The listing builds one solid part. Answer for the finished solid, in the listing's coordinates (mm). A direction names the side the tool comes from. Coordinates: 2 decimals unless noted, no trailing zeros. Order: outer loops, then holes, each group sorted by start corner. A loop starts at its lowest first (then second) coordinate and runs counter-clockwise, first axis right, second up. Notation, with made-up numbers: (39, 48.25) - (90, 48.25) arc R14 cw to (90, 74.25) - close; hole circle Ø11 at (23, 45). An arc over 180 degrees is marked (long way). One line per item, written item: value. Start each with the question number.
```python
from build123d import *

# Parameters (mm, degrees)
SKETCH1_W           = 10
SKETCH1_H           = 26
BOSS_EXTRUDE1_DEPTH = 15
SKETCH2_R           = 5
BOSS_EXTRUDE2_DEPTH = 20


with BuildPart() as part:
    # Sketch1 → Boss-Extrude1 (new body)
    with BuildSketch(Plane.XY):
        Rectangle(SKETCH1_W, SKETCH1_H)
    extrude(amount=BOSS_EXTRUDE1_DEPTH)

    # Sketch2 → Boss-Extrude2 (add)
    with BuildSketch(Plane.XY.offset(15)):
        Circle(SKETCH2_R)
    extrude(amount=BOSS_EXTRUDE2_DEPTH)

    # Sketch3 → Revolve1 (revolve)
    with BuildSketch(Plane.XY.offset(35)):
        with BuildLine():
            Line((-7, 0), (7, 0))
            ThreePointArc((7, 0), (0, 7), (-7, 0))
        make_face()
    revolve(axis=Axis((-7, 0, 35), (1, 0, 0)))


solid = part.part
```
(1) Consider probe 1 along Z at (x, y) = (1.5, -9.5); probe 2 along X at (y, z) = (7.75, 9.5); probe 3 along Z at (x, y) = (-4, 3.25). Determine where each line is inside the solid, lowest interval first.
(2) The part is cut by section B-B on y = -1.75. Determine the outline of the cut face in (x, z).
(3) The part is cut by section C-C on z = 26. Determine the outline of the cut face in (x, y).
(4) Flat-ended cylindrical pins translate along their axes: pin 1 Ø2 at (y, z) = (5, 29) entering from -X; pin 2 Ø5 at (x, y) = (1.5, 6.5) entering from +Z; pin 3 Ø4 at (x, z) = (0, 32) entering from +Y; pin 4 Ø6 at (x, y) = (-1, -0.5) entering from -Z. Find the tip coordinate at first contact, or state that the pin passes through.
(5) For faces 4 (the face through (5, 0, 7)), 5 (the face through (0, 13, 7)), 6 (the face through (-1.08, -4.88, 22.44)), determine the directions among +Z, -Z, +X, -X, +Y, -Y from which every point of the face is accessible in a straight line to the end or side of a thin tool.
(6) The part is cut by section D-D on y = -10.25. Determine the outline of the cut face in (x, z).
(7) The part is cut by section A-A on x = -3. Determine the outline of the cut face in (y, z).
(8) For a pull along Z with two mould halves and no side action, classify faces 1 (the face through (-5, 0, 7)), 2 (the face through (0, 8, 15)), 3 (the face through (0, 0, 0)) as pulls with the +Z half, pulls with the -Z half, needs draft (parallel to the pull), parting line crosses it, or undercut.
Completed:
1. probe 1: z = 0 to 15
1. probe 2: x = -5 to 5
1. probe 3: z = 0 to 15, 30.26 to 39.74
2. outline: (-5, 0) - (5, 0) - (5, 15) - (4.68, 15) - (4.68, 30.1) arc R6.78 ccw (long way) to (-4.68, 30.1) - (-4.68, 15) - (-5, 15) - close
3. outline: circle Ø10 at (0, 0)
4. pin 1: stops at x = -3
4. pin 2: stops at z = 40.62
4. pin 3: stops at y = 6.93
4. pin 4: stops at z = 0
5. face 4: -Z, +X, +Y, -Y
5. face 5: +Z, -Z, +X, -X, +Y
5. face 6: none
6. outline: (-5, 0) - (5, 0) - (5, 15) - (-5, 15) - close
7. outline: (-13, 0) - (13, 0) - (13, 15) - (4, 15) - (4, 30.1) arc R6.32 ccw (long way) to (-4, 30.1) - (-4, 15) - (-13, 15) - close
8. face 1: needs draft
8. face 2: undercut
8. face 3: pulls with the -Z half
